from build123d import *

# Parameters (mm, degrees)
BOSS_EXTRUDE1_DEPTH                = 9.525
F_8_32_TAPPED_HOLE1_D              = 3.4544
F_5_8_0_625_DIAMETER_HOLE1_D       = 15.875
F_6_32_TAPPED_HOLE1_D              = 2.7051
F_6_32_TAPPED_HOLE1_DEPTH          = 8.128
F_6_32_TAPPED_HOLE1_TIP            = 0.81269403
SKETCH8_R                          = 38.1
SKETCH8_R_2                        = 1.35255
SKETCH8_R_3                        = 7.9375
CUT_EXTRUDE1_DEPTH                 = 0.254
F_8_32_TAPPED_HOLE2_D              = 3.4544
F_5_16_0_3125_DIAMETER_HOLE1_D     = 7.9375
F_5_16_0_3125_DIAMETER_HOLE1_DEPTH = 5.08
F_5_16_0_3125_DIAMETER_HOLE1_TIP   = 2.384665582


with BuildPart() as part:
    # Sketch1 → Boss-Extrude1 (new body)
    with BuildSketch(Plane(origin=(0, 0, 0), x_dir=(1, 0, 0), z_dir=(0, 1, 0))):
        Polygon((-96.8375, 122.2375), (-122.2375, 96.8375), (-122.2375, -96.8375), (-96.8375, -122.2375), (96.8375, -122.2375), (122.2375, -96.8375), (122.2375, 96.8375), (96.8375, 122.2375), align=None)
    extrude(amount=BOSS_EXTRUDE1_DEPTH)

    # #8-32 Tapped Hole1 (through all)
    with Locations(Plane(origin=(0, 9.525, 0), x_dir=(1, 0, 0), z_dir=(0, 1, 0))):
        with Locations((-47.0535, 113.6015), (47.0535, 113.6015), (47.0535, -113.6015), (-47.0535, -113.6015)):
            Hole(F_8_32_TAPPED_HOLE1_D / 2)

    # 5/8 (0.625) Diameter Hole1 (through all)
    with Locations(Plane(origin=(0, 9.525, 0), x_dir=(1, 0, 0), z_dir=(0, 1, 0))):
        with Locations((-63.9445, 0)):
            Hole(F_5_8_0_625_DIAMETER_HOLE1_D / 2)

    # #6-32 Tapped Hole1
    with Locations(Plane(origin=(0, 9.525, 0), x_dir=(1, 0, 0), z_dir=(0, 1, 0))):
        with Locations((-78.232, -26.9875), (-49.657, -26.9875), (-49.657, 26.9875), (-78.232, 26.9875)):
            Hole(F_6_32_TAPPED_HOLE1_D / 2, depth=F_6_32_TAPPED_HOLE1_DEPTH)
            with Locations((0, 0, -(F_6_32_TAPPED_HOLE1_DEPTH + F_6_32_TAPPED_HOLE1_TIP / 2))):  # 118° drill point
                Cone(0, F_6_32_TAPPED_HOLE1_D / 2, F_6_32_TAPPED_HOLE1_TIP, mode=Mode.SUBTRACT)

    # Sketch8 → Cut-Extrude1 (cut)
    with BuildSketch(Plane(origin=(0, 9.525, 0), x_dir=(1, 0, 0), z_dir=(0, 1, 0))):
        with Locations(Location((-63.9445, 0, 0), (0, 0, 270))):  # turned: the seam where the file's is
            Circle(SKETCH8_R)
        with Locations(Location((-78.232, -26.9875, 0), (0, 0, 270))):  # turned: the seam where the file's is
            Circle(SKETCH8_R_2, mode=Mode.SUBTRACT)
        with Locations(Location((-49.657, 26.9875, 0), (0, 0, 270))):  # turned: the seam where the file's is
            Circle(SKETCH8_R_2, mode=Mode.SUBTRACT)
        with Locations(Location((-63.9445, 0, 0), (0, 0, 270))):  # turned: the seam where the file's is
            Circle(SKETCH8_R_3, mode=Mode.SUBTRACT)
        with Locations(Location((-78.232, 26.9875, 0), (0, 0, 270))):  # turned: the seam where the file's is
            Circle(SKETCH8_R_2, mode=Mode.SUBTRACT)
        with Locations(Location((-49.657, -26.9875, 0), (0, 0, 270))):  # turned: the seam where the file's is
            Circle(SKETCH8_R_2, mode=Mode.SUBTRACT)
    extrude(amount=-CUT_EXTRUDE1_DEPTH, mode=Mode.SUBTRACT)

    # #8-32 Tapped Hole2 (through all)
    with Locations(Plane(origin=(0, 9.525, 0), x_dir=(1, 0, 0), z_dir=(0, 1, 0))):
        with Locations((-103.1875, 103.1875), (103.1875, 103.1875), (103.1875, -103.1875), (-103.1875, -103.1875)):
            Hole(F_8_32_TAPPED_HOLE2_D / 2)

    # 5/16 (0.3125) Diameter Hole1
    with Locations(Plane(origin=(0, 0, 0), x_dir=(-1, 0, 0), z_dir=(0, -1, 0))):
        with Locations((85.0011, 0), (-85.0011, -52.5145), (-85.0011, 52.4891)):
            Hole(F_5_16_0_3125_DIAMETER_HOLE1_D / 2, depth=F_5_16_0_3125_DIAMETER_HOLE1_DEPTH)
            with Locations((0, 0, -(F_5_16_0_3125_DIAMETER_HOLE1_DEPTH + F_5_16_0_3125_DIAMETER_HOLE1_TIP / 2))):  # 118° drill point
                Cone(0, F_5_16_0_3125_DIAMETER_HOLE1_D / 2, F_5_16_0_3125_DIAMETER_HOLE1_TIP, mode=Mode.SUBTRACT)


solid = part.part
The model under review builds one solid part; all positions refer to its coordinate system, in mm. A direction names the side the tool comes from. Round coordinates to 2 decimals unless told otherwise and drop trailing zeros. Write item = value, one per line. Start each with the question number.
Item 1: For faces 1 (the flat face through (-72, 9.271, -1)), 2 (the cylindrical face through (82.1, 2.6, -55.2)), 3 (the flat face through (-109.715, 4.696, 109.36)), list the 3-axis set-ups (+Z, -Z, +X, -X, +Y, -Y) from which the entire face can be reached by the end or side of a thin tool; tool diameter is ignored.
Item 2: Mouldability with a two-part tool opening along X and no side actions: class faces 4 (the cylindrical face through (-88.966, 2.576, -0.174)), 5 (the flat face through (-122.238, 5, -1)), 6 (the flat face through (109.715, 4.696, -109.36)) as released by +X, released by -X, zero draft, split by the parting line, or undercut.
Item 3: Insertion check: pin 1 (3 mm diameter, centred on x = -103.19, z = -103.19, fed in from +Y); pin 2 (3 mm diameter, centred on x = -49.66, z = 26.99, fed in from +Y). Each pin has a flat end and moves straight along its axis. Give the tip position at first contact, or say it passes through.
Item 4: To check wall thickness, follow L1, parallel to X at y = 9.4, z = 0; L2, parallel to Z at x = -102.5, y = 8.5 (3 decimals); L3, parallel to Z at x = 48.5, y = 2.5. State the ranges of each line that lie inside material, in increasing order.
Item 5: Take a section at A-A on y = 3. Count the separate pieces of the cut face and the enclosed holes in it, plus the area to 3 significant figures.
Result:
q1.face_1 = +Y
q1.face_2 = -Y
q1.face_3 = +Z, -X, +Y, -Y
q2.face_4 = undercut
q2.face_5 = released by -X
q2.face_6 = released by +X
q3.pin_1 = through
q3.pin_2 = 9.27
q4.L1 = -122.24 to -102.04, -25.84 to 122.24
q4.L2 = -116.575 to -104.772, -101.603 to 101.603, 104.772 to 116.575
q4.L3 = -122.24 to -114.55, -112.66 to 112.66, 114.55 to 122.24
q5.separate_pieces = 1
q5.enclosed_holes = 16
q5.area = 58,000 mm²
